Verification items for the finished model (mm, model axes). Face numbers are marked on the shaded views. A direction names the side the tool comes from. Round coordinates to 2 decimals unless told otherwise and drop trailing zeros. Write each loop counter-clockwise with the first axis right and the second up, starting at its lowest first coordinate (ties: lowest second). Pieces come first, ordered by that corner, then holes. Notation, with made-up numbers: (53, -14) -> (79, -14) arc R12 ccw to (79, 9) -> close; hole circle Ø1 at (-34.5, 89.25). An arc over 180 degrees is marked (long way). Use CSV: the item, a comma, the result in double quotes.
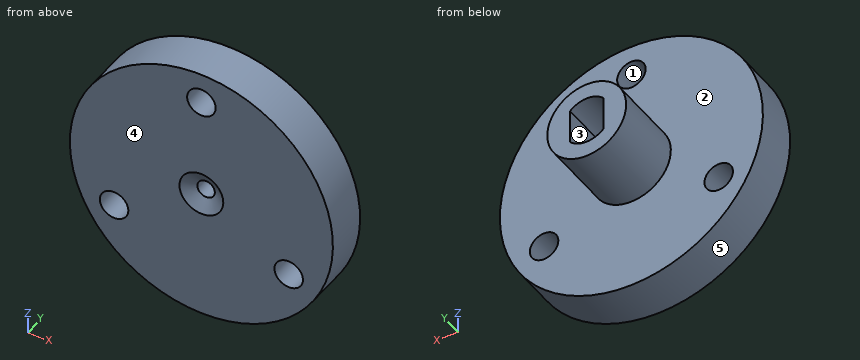
```python
from build123d import *

# Parameters (mm, degrees)
SKETCH1_R           = 4.5
BOSS_EXTRUDE1_DEPTH = 8.2
SKETCH2_R           = 15
BOSS_EXTRUDE2_DEPTH = 5
SKETCH3_R           = 1
CUT_EXTRUDE1_DEPTH  = 25.984795376
SKETCH4_R           = 1.625
CUT_EXTRUDE2_DEPTH  = 25.984795376
CHAMFER1_SIZE       = 1.5
CHAMFER1_SIZE2      = 0.866025404


with BuildPart() as part:
    # Sketch1 → Boss-Extrude1 (new body)
    with BuildSketch(Plane(origin=(0, 0, 0), x_dir=(1, 0, 0), z_dir=(0, 1, 0))):
        with Locations(Location((0, 0, 0), (0, 0, 270))):
            Circle(SKETCH1_R)
        with BuildLine():
            Line((-1.9, 1.953362486), (-1.9, -1.953362486))
            ThreePointArc((-1.9, -1.953362486), (0, -2.725), (1.9, -1.953362486))
            Line((1.9, -1.953362486), (1.9, 1.953362486))
            ThreePointArc((1.9, 1.953362486), (0, 2.725), (-1.9, 1.953362486))
        make_face(mode=Mode.SUBTRACT)
    extrude(amount=BOSS_EXTRUDE1_DEPTH)

    # Sketch2 → Boss-Extrude2 (add)
    with BuildSketch(Plane.XZ):
        with Locations(Location((0, 0, 0), (0, 0, 270))):
            Circle(SKETCH2_R)
    extrude(amount=BOSS_EXTRUDE2_DEPTH)

    # Sketch3 → Cut-Extrude1 (cut, through all)
    with BuildSketch(Plane.XZ.offset(5)):
        with Locations(Location((0, 0, 0), (0, 0, 270))):
            Circle(SKETCH3_R)
    extrude(amount=-CUT_EXTRUDE1_DEPTH, mode=Mode.SUBTRACT)

    # Sketch4 → Cut-Extrude2 (cut, through all)
    with BuildSketch(Plane.XZ.offset(5)):
        with Locations(Location((0, 11.5, 0), (0, 0, 270))):
            Circle(SKETCH4_R)
        with Locations(Location((9.959292144, -5.75, 0), (0, 0, 270))):
            Circle(SKETCH4_R)
        with Locations(Location((-9.959292144, -5.75, 0), (0, 0, 270))):
            Circle(SKETCH4_R)
    extrude(amount=-CUT_EXTRUDE2_DEPTH, mode=Mode.SUBTRACT)

    # Chamfer1
    chamfer1_edges = [part.edges().sort_by_distance(p)[0] for p in [
        (0, -5, 1),
    ]]
    chamfer1_side = [part.faces().sort_by_distance(p)[0] for p in [
        (0, -5, 14.575735931),
    ]]
    chamfer(chamfer1_edges, length=CHAMFER1_SIZE, length2=CHAMFER1_SIZE2, reference=chamfer1_side[0])


solid = part.part
```
Q1. Section check B-B (y = 1.5). Record the cut outline in (x, z) (3 decimals).
Filled in:
outline,"circle Ø9 at (0, 0); hole (-1.9, -1.953) arc R2.725 ccw to (1.9, -1.953) -> (1.9, 1.953) arc R2.725 ccw to (-1.9, 1.953) -> close"
Q2. Access from +Z, -Z, +X, -X, +Y, -Y to the whole of each face (thin tool, end or side, straight path). Record for the marked faces 1 and 2.
Filled in:
face 1,"+Y, -Y"
face 2,"+Y"
Q3. Section check D-D (y = -3.25). Record the cut outline in (x, z) (3 decimals).
Filled in:
outline,"circle Ø30 at (0, 0); hole circle Ø3.25 at (-9.959, -5.75); hole circle Ø3.25 at (0, 11.5); hole circle Ø2 at (0, 0); hole circle Ø3.25 at (9.959, -5.75)"
Q4. Go/stop test with flat-tipped pins: P1, Ø5, axis at y = -0.5, z = -5.5, coming from the -X side; P2, Ø3, axis at x = -5, z = -8, coming from the +Y side; P3, Ø3, axis at y = 3, z = 0, coming from the +X side. Record where each tip stops, or that it passes through.
Filled in:
P1,"x = -14.7"
P2,"y = 0"
P3,"x = 4.5"
Q5. Section check C-C (z = -5.75). Record the cut outline in (x, y), plus the area to 3 significant figures.
Filled in:
outline,"(-13.85, -5) -> (-11.58, -5) -> (-11.58, 0) -> (-13.85, 0) -> close; (-8.33, -5) -> (8.33, -5) -> (8.33, 0) -> (-8.33, 0) -> close; (11.58, -5) -> (13.85, -5) -> (13.85, 0) -> (11.58, 0) -> close"
area,"106 mm²"
Q6. Material ranges on L1, parallel to X at y = -1.3, z = 0; L2, parallel to Y at x = -11, z = 3.25; L3, parallel to X at y = -2.8, z = 11.5 (3 decimals), recorded low to high.
Filled in:
L1,"-15 to -1, 1 to 15"
L2,"-5 to 0"
L3,"-9.631 to -1.625, 1.625 to 9.631"
Q7. Section check A-A (z = 0). Record the cut outline in (x, y).
Filled in:
outline,"(-15, -5) -> (-2.5, -5) -> (-1, -4.13) -> (-1, 0) -> (-1.9, 0) -> (-1.9, 8.2) -> (-4.5, 8.2) -> (-4.5, 0) -> (-15, 0) -> close; (1, -4.13) -> (2.5, -5) -> (15, -5) -> (15, 0) -> (4.5, 0) -> (4.5, 8.2) -> (1.9, 8.2) -> (1.9, 0) -> (1, 0) -> close"
Q8. Mould release check, pull along X, two halves, no side actions. Record for the marked faces 3, 4 and 5: released by +X, released by -X, zero draft, split by the parting line, or undercut.
Filled in:
face 3,"undercut"
face 4,"zero draft"
face 5,"split by the parting line"
